Could you check a few things on this model? Use its own coordinates, in mm. Face numbers are marked on the shaded views. A direction names the side the tool comes from. Give positions to 0.01 mm unless a question says otherwise; leave off trailing zeros. Loops run counter-clockwise (first coordinate to the right, second up) from the corner with the lowest first, then second, coordinate; pieces in that order, holes last. Notation, with made-up numbers: M -3.5,11 L 7.5,11 A21 cw 7.5,31 Z; hole C 32,-4.5 d9. An arc over 180 degrees is marked long. Use a Markdown table: item, result. Add a question column.
1) Will these pins go through, and if not, where does the flat tip stop? pin 1 Ø2 at (y, z) = (6, -2.5) entering from -X; pin 2 Ø3 at (x, y) = (2, 4.5) entering from -Z; pin 3 Ø1.3 at (x, z) = (0, -0.5) entering from -Y.
2) We'd pull the mould along X, two halves only. Please class the marked faces 4, 5, 6 and 7: +X half, -X half, draft (parallel to the pull), parting line (faces both ways), or undercut.
3) Suppose I cut it at A-A on x = 0. List the corners of the cut face in (y, z) for me.
4) Which directions (+Z, -Z, +X, -X, +Y, -Y) give clear straight access to the entire face, cutting with the end or side of a thin tool? Please do the marked faces 1, 2 and 3.
5) Suppose I cut it at D-D on y = 3.25. List the corners of the cut face in (x, z) for me.
6) If I drill on line 1 along X through (y, z) = (0.5, 0); line 2 along Y through (x, z) = (0.75, -1.25); line 3 along Z through (x, y) = (-1, 0.5), over which ranges is the centre line in solid material (lowest first)? Write a range as [from, to].
7) Suppose I cut it at C-C on y = 1.25. List the corners of the cut face in (x, z) for me, and give its area (3 significant figures).
8) Suppose I cut it at B-B on z = 0. List the corners of the cut face in (x, y) for me.
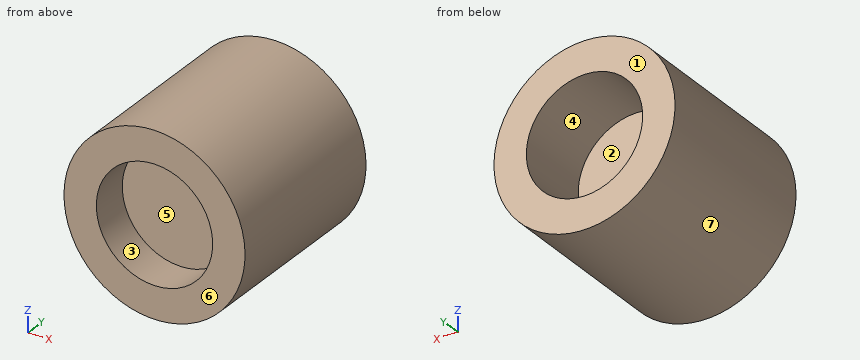
```python
from build123d import *

# Parameters (mm, degrees)
CROQUIS1_R              = 3.5
SALIENTE_EXTRUIR1_DEPTH = 7
CROQUIS2_R              = 2.25
CORTAR_EXTRUIR1_DEPTH   = 3
CORTAR_EXTRUIR2_START   = -1.5
CROQUIS3_R              = 2.25
CORTAR_EXTRUIR2_DEPTH   = 1.5


with BuildPart() as part:
    # Croquis1 → Saliente-Extruir1 (new body)
    with BuildSketch(Plane(origin=(0, 0, 0), x_dir=(1, 0, 0), z_dir=(0, 1, 0))):
        with Locations(Location((0, 0, 0), (0, 0, 270))):
            Circle(CROQUIS1_R)
    extrude(amount=SALIENTE_EXTRUIR1_DEPTH)

    # Croquis2 → Cortar-Extruir1 (cut)
    with BuildSketch(Plane(origin=(0, 7, 0), x_dir=(1, 0, 0), z_dir=(0, 1, 0))):
        with Locations(Location((0, 0, 0), (0, 0, 270))):
            Circle(CROQUIS2_R)
    extrude(amount=-CORTAR_EXTRUIR1_DEPTH, mode=Mode.SUBTRACT)

    # Croquis3 → Cortar-Extruir2 (cut)
    with BuildSketch(Plane.XZ.offset(CORTAR_EXTRUIR2_START)):
        with Locations(Location((0, 0, 0), (0, 0, 90))):
            Circle(CROQUIS3_R)
    extrude(amount=CORTAR_EXTRUIR2_DEPTH, mode=Mode.SUBTRACT)


solid = part.part
```
Answer block:
| question | item | result |
|---|---|---|
| 1 | pin 1 | stops at x = -3.16 |
| 1 | pin 2 | stops at z = -3.46 |
| 1 | pin 3 | stops at y = 1.5 |
| 2 | face 4 | undercut |
| 2 | face 5 | undercut |
| 2 | face 6 | draft |
| 2 | face 7 | parting line |
| 3 | outline | M 0,-3.5 L 7,-3.5 L 7,-2.25 L 4,-2.25 L 4,2.25 L 7,2.25 L 7,3.5 L 0,3.5 L 0,2.25 L 1.5,2.25 L 1.5,-2.25 L 0,-2.25 Z |
| 4 | face 1 | +Z, -Z, +X, -X, +Y |
| 4 | face 2 | +Y |
| 4 | face 3 | -Y |
| 5 | outline | C 0,0 d7 |
| 6 | line 1 | x = [-3.5, -2.25], [2.25, 3.5] |
| 6 | line 2 | y = [1.5, 4] |
| 6 | line 3 | z = [-3.35, -2.02], [2.02, 3.35] |
| 7 | outline | C 0,0 d7; hole C 0,0 d4.5 |
| 7 | area | 22.6 mm^2 |
| 8 | outline | M -3.5,0 L -2.25,0 L -2.25,1.5 L 2.25,1.5 L 2.25,0 L 3.5,0 L 3.5,7 L 2.25,7 L 2.25,4 L -2.25,4 L -2.25,7 L -3.5,7 Z |
